Design review of the part built by this model. Coordinates are the model's own, in mm. Face numbers are marked on the shaded views. A direction names the side the tool comes from. Give positions to 0.01 mm unless a question says otherwise; leave off trailing zeros. Write each loop counter-clockwise with the first axis right and the second up, starting at its lowest first coordinate (ties: lowest second). Pieces come first, ordered by that corner, then holes.
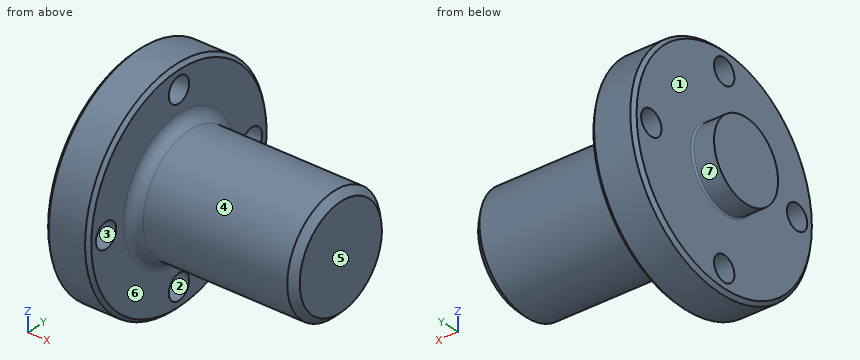
```python
from build123d import *

# Parameters (mm, degrees)
SKETCH1_R           = 24.6126
BOSS_EXTRUDE1_DEPTH = 9.525
BOSS_EXTRUDE2_START = 9.525
SKETCH2_R           = 12.7
BOSS_EXTRUDE2_DEPTH = 35.7124
SKETCH3_R           = 8.7122
BOSS_EXTRUDE4_DEPTH = 4.826
SKETCH4_R           = 2.7686
CUT_EXTRUDE2_DEPTH  = 58.078739617
FILLET1_R           = 0.381
FILLET2_R           = 2.3876
CHAMFER1_SIZE       = 0.762
CHAMFER2_SIZE       = 1.524


with BuildPart() as part:
    # Sketch1 → Boss-Extrude1 (new body)
    with BuildSketch(Plane.YZ):
        with Locations(Location((0, 0, 0), (0, 0, 270))):
            Circle(SKETCH1_R)
    extrude(amount=BOSS_EXTRUDE1_DEPTH)

    # Sketch2 → Boss-Extrude2 (add)
    with BuildSketch(Plane.YZ.offset(BOSS_EXTRUDE2_START)):
        with Locations(Location((0, 0, 0), (0, 0, 270))):
            Circle(SKETCH2_R)
    extrude(amount=BOSS_EXTRUDE2_DEPTH)

    # Sketch3 → Boss-Extrude4 (add)
    with BuildSketch(Plane.YZ):
        with Locations(Location((0, 0, 0), (0, 0, 270))):
            Circle(SKETCH3_R)
    extrude(amount=-BOSS_EXTRUDE4_DEPTH)

    # Sketch4 → Cut-Extrude2 (cut, through all)
    with BuildSketch(Plane.YZ):
        with Locations(Location((0, 19.8374, 0), (0, 0, 270))):
            Circle(SKETCH4_R)
        with Locations(Location((19.8374, 0, 0), (0, 0, 270))):
            Circle(SKETCH4_R)
        with Locations(Location((0, -19.8374, 0), (0, 0, 270))):
            Circle(SKETCH4_R)
        with Locations(Location((-19.8374, 0, 0), (0, 0, 270))):
            Circle(SKETCH4_R)
    extrude(amount=CUT_EXTRUDE2_DEPTH, mode=Mode.SUBTRACT)

    # Fillet1
    fillet1_edges = [part.edges().sort_by_distance(p)[0] for p in [
        (0, 0, 8.7122),
    ]]
    fillet(fillet1_edges, radius=FILLET1_R)

    # Fillet2
    fillet2_edges = [part.edges().sort_by_distance(p)[0] for p in [
        (9.525, 0, 12.7),
    ]]
    fillet(fillet2_edges, radius=FILLET2_R)

    # Chamfer1
    chamfer1_edges = [part.edges().sort_by_distance(p)[0] for p in [
        (0, 0, 24.6126),
        (9.525, 0, 24.6126),
    ]]
    chamfer(chamfer1_edges, length=CHAMFER1_SIZE)

    # Chamfer2
    chamfer2_edges = [part.edges().sort_by_distance(p)[0] for p in [
        (45.2374, 0, 12.7),
    ]]
    chamfer(chamfer2_edges, length=CHAMFER2_SIZE)


solid = part.part
```
(1) Clearance check with flat-ended pins moving along their axes: P1, Ø2, axis at x = 22.5, z = 7, coming from the -Y side; P2, Ø1, axis at y = -8, z = -14.5, coming from the -X side; P3, Ø1, axis at x = 35.5, y = 3.5, coming from the +Z side. State where each tip first meets the part, or that it passes through.
Resolved:
P1: stops at y = -11.19
P2: stops at x = 0
P3: stops at z = 12.34
(2) Tool access review of the marked faces 5, 6 and 7: name each direction out of +Z, -Z, +X, -X, +Y, -Y from which nothing blocks a thin tool from reaching the whole face with its end or side.
Resolved:
face 5: +Z, -Z, +X, +Y, -Y
face 6: +X
face 7: -X
(3) Mouldability with a two-part tool opening along Y and no side actions: class the marked faces 1, 2, 3 and 4 as pulls with the +Y half, pulls with the -Y half, needs draft (parallel to the pull), parting line crosses it, or undercut.
Resolved:
face 1: needs draft
face 2: undercut
face 3: undercut
face 4: parting line crosses it
(4) Consider section C-C, the plane x = 37. Give the boundary of the cut face in (y, z), then the cut area to 3 significant figures.
Resolved:
outline: circle Ø25.4 at (0, 0)
area: 507 mm2
(5) To check wall thickness, follow L1, parallel to Y at x = 2, z = 0; L2, parallel to X at y = 15.5, z = 5.5 (3 decimals); L3, parallel to Y at x = 5.5, z = -19.5. State the ranges of each line that lie inside material, in increasing order.
Resolved:
L1: y = -24.61 to -22.61, -17.07 to 17.07, 22.61 to 24.61
L2: x = 0 to 9.525
L3: y = -15.02 to -2.75, 2.75 to 15.02
(6) Consider section A-A, the plane y = 0. Give the number of separate pieces and of enclosed holes in the cut face, then the cut area to 3 significant figures.
Resolved:
separate pieces: 3
enclosed holes: 0
area: 1,350 mm2
